from build123d import *

# Parameters (mm, degrees)
SKETCH2_W                       = 8
SKETCH2_H                       = 2
BOSS_EXTRUDE1_REACH             = 42.128
SKETCH3_R                       = 1.5
BOSS_EXTRUDE1_DIRECTION_2_REACH = 42.128
BOSS_EXTRUDE2_DEPTH             = 5
FILLET1_R                       = 1
FILLET2_R                       = 1
CIRPATTERN1_COUNT               = 5
FILLET1_OF_CIRPATTERN1_R        = 1
FILLET2_OF_CIRPATTERN1_R        = 1
BOSS_EXTRUDE3_START             = 3
BOSS_EXTRUDE3_DEPTH             = 3
FILLET3_R                       = 0.5


with BuildPart() as part:
    # Sketch2 → Revolve1 (revolve)
    with BuildSketch(Plane.XY):
        with Locations((0, -24)):
            Rectangle(SKETCH2_W, SKETCH2_H)
        with BuildLine():
            Line((2.5, -25), (-2.5, -25))
            Line((-2.5, -25), (-2.5, -27.5))
            ThreePointArc((-2.5, -27.5), (-2.353553391, -27.853553391), (-2, -28))
            Line((-2, -28), (2, -28))
            ThreePointArc((2, -28), (2.353553391, -27.853553391), (2.5, -27.5))
            Line((2.5, -27.5), (2.5, -25))
        make_face()
    revolve(axis=Axis((-65.527863449, 0, 0), (1, 0, 0)))


with BuildPart() as body_2:

    # Boss-Extrude1: up to this face of the body (flat: up to its plane)
    boss_extrude1_end = Plane(part.part.faces().sort_by_distance((4, 24.292893219, 0))[0])
    # Sketch3 → Boss-Extrude1 (new, up to the picked face)
    with BuildSketch(Plane.ZY.offset(2.5), mode=Mode.PRIVATE) as boss_extrude1_sk1:
        with BuildLine():
            Line((-1.109469632, 1.009493505), (1.109469632, 1.009493505))
            ThreePointArc((1.109469632, 1.009493505), (1.455460496, -0.362815028), (0.505806645, -1.412147173))
            Line((0.505806645, -1.412147173), (0.505806645, -9.597975753))
            ThreePointArc((0.505806645, -9.597975753), (0, 9.611294342), (-0.505806645, -9.597975753))
            Line((-0.505806645, -9.597975753), (-0.505806645, -1.412147173))
            ThreePointArc((-0.505806645, -1.412147173), (-1.455460496, -0.362815028), (-1.109469632, 1.009493505))
        make_face()
        with Locations(Location((6.35, 0, 0), (0, 0, 90))):
            Circle(SKETCH3_R, mode=Mode.SUBTRACT)
        with Locations(Location((-6.35, 0, 0), (0, 0, 90))):
            Circle(SKETCH3_R, mode=Mode.SUBTRACT)
    boss_extrude1_tool1 = split(extrude(boss_extrude1_sk1.sketch, amount=-BOSS_EXTRUDE1_REACH, mode=Mode.PRIVATE), bisect_by=boss_extrude1_end, keep=Keep.BOTH, mode=Mode.PRIVATE)
    add(boss_extrude1_tool1.solids().sort_by(Axis((-2.5, 1.281248, 0), (1, 0, 0)))[0])


    # Boss-Extrude1 direction 2: up to this face of the body (flat: up to its plane)
    boss_extrude1_direction_2_end = Plane(part.part.faces().sort_by_distance((-4, 23.707106781, 0))[0])
    # Sketch3 → Boss-Extrude1 direction 2 (add, up to the picked face)
    with BuildSketch(Plane.ZY.offset(2.5), mode=Mode.PRIVATE) as boss_extrude1_direction_2_sk1:
        with BuildLine():
            Line((-1.109469632, 1.009493505), (1.109469632, 1.009493505))
            ThreePointArc((1.109469632, 1.009493505), (1.455460496, -0.362815028), (0.505806645, -1.412147173))
            Line((0.505806645, -1.412147173), (0.505806645, -9.597975753))
            ThreePointArc((0.505806645, -9.597975753), (0, 9.611294342), (-0.505806645, -9.597975753))
            Line((-0.505806645, -9.597975753), (-0.505806645, -1.412147173))
            ThreePointArc((-0.505806645, -1.412147173), (-1.455460496, -0.362815028), (-1.109469632, 1.009493505))
        make_face()
        with Locations(Location((6.35, 0, 0), (0, 0, 90))):
            Circle(SKETCH3_R, mode=Mode.SUBTRACT)
        with Locations(Location((-6.35, 0, 0), (0, 0, 90))):
            Circle(SKETCH3_R, mode=Mode.SUBTRACT)
    boss_extrude1_direction_2_tool1 = split(extrude(boss_extrude1_direction_2_sk1.sketch, amount=BOSS_EXTRUDE1_DIRECTION_2_REACH, mode=Mode.PRIVATE), bisect_by=boss_extrude1_direction_2_end, keep=Keep.BOTH, mode=Mode.PRIVATE)
    add(boss_extrude1_direction_2_tool1.solids().sort_by(Axis((-2.5, 1.281248, 0), (-1, 0, 0)))[0])


with BuildPart() as part_1:
    add(part.part)

    add(body_2.part)  # Boss-Extrude2 merges body 2
    # Sketch4 → Boss-Extrude2 (add)
    with BuildSketch(Plane.ZY.offset(2.5)):
        with BuildLine():
            Line((2.193830501, 9.357568416), (1.783681385, 22.930732232))
            ThreePointArc((1.783681385, 22.930732232), (0, 23), (-1.783681385, 22.930732232))
            Line((-1.783681385, 22.930732232), (-2.193830501, 9.357568416))
            ThreePointArc((-2.193830501, 9.357568416), (0, 9.611294342), (2.193830501, 9.357568416))
        make_face()
        with BuildLine():
            ThreePointArc((-1.15, 11.702139555), (0, 11.332236709), (1.15, 11.702139555))
            Line((1.15, 11.702139555), (0.86465248, 21.14521399))
            ThreePointArc((0.86465248, 21.14521399), (0.713053714, 21.488965069), (0.364880601, 21.630112058))
            Line((0.364880601, 21.630112058), (-0.364880601, 21.630112058))
            ThreePointArc((-0.364880601, 21.630112058), (-0.713053714, 21.488965069), (-0.86465248, 21.14521399))
            Line((-0.86465248, 21.14521399), (-1.15, 11.702139555))
        make_face(mode=Mode.SUBTRACT)
    boss_extrude2 = extrude(amount=-BOSS_EXTRUDE2_DEPTH)

    # Fillet1
    fillet1_edges = [part_1.edges().sort_by_distance(p)[0] for p in [
        (0, 22.930732232, 1.783681385),
    ]]
    fillet(fillet1_edges, radius=FILLET1_R)

    # Fillet2
    fillet2_edges = [part_1.edges().sort_by_distance(p)[0] for p in [
        (0, 22.930732232, -1.783681385),
    ]]
    fillet(fillet2_edges, radius=FILLET2_R)

    # CirPattern1: Boss-Extrude2 ×5 about axis
    cirpattern1_axis = Axis((0, 0, 0), (1, 0, 0))
    for i in range(1, CIRPATTERN1_COUNT):
        add(boss_extrude2.rotate(cirpattern1_axis, i * 360 / CIRPATTERN1_COUNT))

    # Fillet1 of CirPattern1
    fillet1_of_cirpattern1_edges = [part_1.edges().sort_by_distance(p)[0] for p in [
        (0, 5.389604149, 22.359610174),
        (0, -19.599773683, 12.035317677),
        (0, -17.502930456, -14.921374784),
        (0, 8.782367758, -21.257234453),
    ]]
    fillet(fillet1_of_cirpattern1_edges, radius=FILLET1_OF_CIRPATTERN1_R)

    # Fillet2 of CirPattern1
    fillet2_of_cirpattern1_edges = [part_1.edges().sort_by_distance(p)[0] for p in [
        (0, 8.782367758, 21.257234453),
        (0, -17.502930456, 14.921374784),
        (0, -19.599773683, -12.035317677),
        (0, 5.389604149, -22.359610174),
    ]]
    fillet(fillet2_of_cirpattern1_edges, radius=FILLET2_OF_CIRPATTERN1_R)

    # Sketch5 → Boss-Extrude3 (add)
    with BuildSketch(Plane.ZY.offset(4).offset(BOSS_EXTRUDE3_START)):
        with BuildLine():
            Line((-1.109469632, 1.009493505), (1.109469632, 1.009493505))
            ThreePointArc((1.109469632, 1.009493505), (1.455460496, -0.362815028), (0.505806645, -1.412147173))
            Line((0.505806645, -1.412147173), (0.505806645, -3.463258529))
            ThreePointArc((0.505806645, -3.463258529), (0, 3.5), (-0.505806645, -3.463258529))
            Line((-0.505806645, -3.463258529), (-0.505806645, -1.412147173))
            ThreePointArc((-0.505806645, -1.412147173), (-1.455460496, -0.362815028), (-1.109469632, 1.009493505))
        make_face()
    extrude(amount=-BOSS_EXTRUDE3_DEPTH)

    # Fillet3
    fillet3_edges = [part_1.edges().sort_by_distance(p)[0] for p in [
        (-7, 3.5, 0),
    ]]
    fillet(fillet3_edges, radius=FILLET3_R)


solid = part_1.part
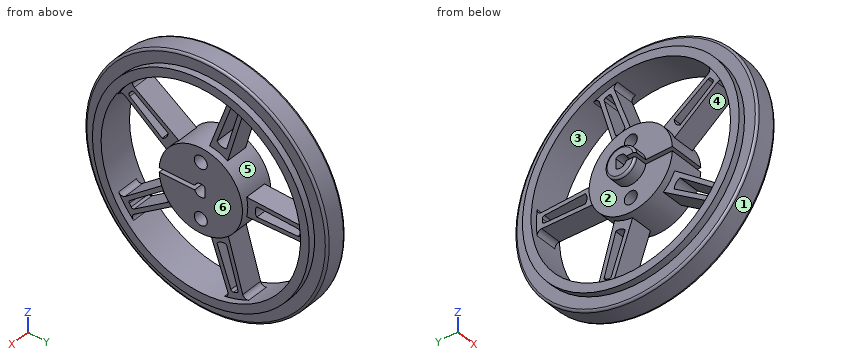
The listing builds one solid part. Answer for the finished solid, in the listing's coordinates (mm). Face numbers are marked on the shaded views. A direction names the side the tool comes from. Coordinates: 2 decimals unless noted, no trailing zeros. One line per question, with ' | ' between items.
1. Which of the six approach directions +Z, -Z, +X, -X, +Y, -Y give full straight-line access (tool end or side, diameter ignored) to the marked faces 4, 5 and 6?
Verdict:
face 4: +X, -X | face 5: none | face 6: +Z, -Z, +X, +Y, -Y
2. Section A-A (y = 0) is taken. State how many separate pieces and enclosed holes the cut face has, and give its area (3 significant figures).
Verdict:
separate pieces: 6 | enclosed holes: 0 | area: 155 mm^2
3. For a pull along Y with two mould halves and no side action, classify the marked faces 1, 2 and 3 as released by +Y, released by -Y, zero draft, split by the parting line, or undercut.
Verdict:
face 1: split by the parting line | face 2: zero draft | face 3: undercut
4. Given pin 1 Ø4 at (x, y) = (-3.5, 12.5) entering from +Z; pin 2 Ø2 at (y, z) = (-18, 18) entering from -X; pin 3 Ø4.5 at (y, z) = (4, -16.5) entering from +X, each flat-ended and moving along its own axis, determine where each tip first touches the part or whether it passes through.
Verdict:
pin 1: stops at z = 25.71 | pin 2: stops at x = -4 | pin 3: stops at x = 2.5
5. Straight lines are drawn through the part: line 1 (Z direction, x = -0.5, y = 0); line 2 (Y direction, x = 1.25, z = 6.35); line 3 (Y direction, x = -1, z = -3.5). For each, find the intervals that lie inside material, in ascending order.
Verdict:
line 1: z = -28 to -23, -9.61 to -7.85, -4.85 to -1.5, 1.5 to 4.85, 7.85 to 9.61, 23 to 28 | line 2: y = -27.27 to -22.11, -12.25 to -10.66, -9.45 to -1.5, 1.5 to 7.21, 22.11 to 27.27 | line 3: y = -27.78 to -22.73, -8.95 to 8.95, 22.73 to 27.78
